The listing builds one solid part. Answer for the finished solid, in the listing's coordinates (mm). Give positions to 0.01 mm unless a question says otherwise; leave off trailing zeros. Order: outer loops, then holes, each group sorted by start corner. A loop starts at its lowest first (then second) coordinate and runs counter-clockwise, first axis right, second up.
```python
from build123d import *

# Parameters (mm, degrees)
SKETCH093_W           = 21
SKETCH093_H           = 96
EXTRUDE085_DEPTH      = 1
SKETCH140_R           = 15
EXTRUDE130_DEPTH      = 3
EXTRUDE130_DEPTH_BACK = 1
EXTRUDE074_DEPTH      = 2


with BuildPart() as cutout:
    # Sketch093 → Extrude085 (new body)
    with BuildSketch(Plane(origin=(0, 0, -25), x_dir=(1, 0, 0), z_dir=(0, 0, -1))):
        with Locations((153, -47.5)):
            Rectangle(SKETCH093_W, SKETCH093_H)
    extrude(amount=EXTRUDE085_DEPTH)


with BuildPart() as compound029:
    # Sketch140 → Extrude130 (new body, two sides)
    with BuildSketch(Plane(origin=(0, 0, -25), x_dir=(1, 0, 0), z_dir=(0, 0, -1))) as extrude130_sk:
        with Locations((25, -27)):
            Circle(SKETCH140_R)
        with Locations((103, -27)):
            Circle(SKETCH140_R)
        with Locations((64, -27)):
            Circle(SKETCH140_R)
        with Locations((103, -71)):
            Circle(SKETCH140_R)
        with Locations((25, -71)):
            Circle(SKETCH140_R)
        with Locations((64, -71)):
            Circle(SKETCH140_R)
        with Locations((188, -30)):
            Circle(SKETCH140_R)
        with Locations((231, -30)):
            Circle(SKETCH140_R)
        with Locations((188, -71)):
            Circle(SKETCH140_R)
        with Locations((231, -71)):
            Circle(SKETCH140_R)
        with Locations((284, -30)):
            Circle(SKETCH140_R)
        with Locations((329, -30)):
            Circle(SKETCH140_R)
        with Locations((284, -71)):
            Circle(SKETCH140_R)
        with Locations((329, -71)):
            Circle(SKETCH140_R)
    extrude(amount=EXTRUDE130_DEPTH)
    extrude(extrude130_sk.sketch, amount=-EXTRUDE130_DEPTH_BACK)

    # Compound029: union cutout
    add(cutout.part)


with BuildPart() as panel002:
    # Sketch082 → Extrude074 (new body)
    with BuildSketch(Plane(origin=(0, 0, -25), x_dir=(1, 0, 0), z_dir=(0, 0, -1))):
        Polygon((-2.5, 1.5), (360.5, 1.5), (360.5, -96.5), (309.5, -96.5), (309.5, -99), (257, -99), (257, -96.5), (205.5, -96.5), (205.5, -99), (153, -99), (153, -96.5), (101.5, -96.5), (101.5, -99), (49, -99), (49, -96.5), (-2.5, -96.5), align=None)
    extrude(amount=EXTRUDE074_DEPTH)

    # Cut: cut Compound029
    add(compound029.part, mode=Mode.SUBTRACT)


solid = panel002.part
```
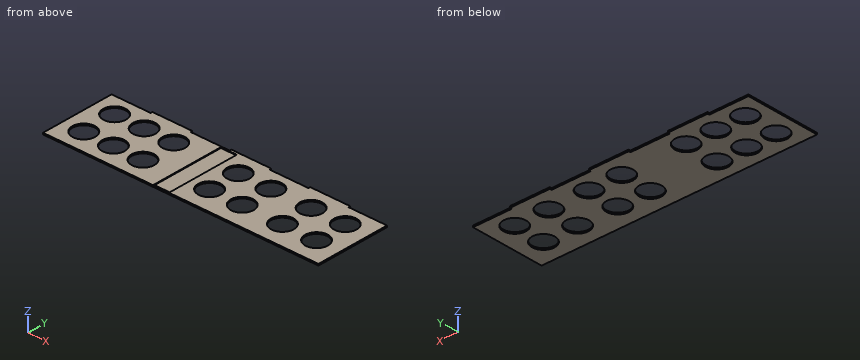
1) Find section D-D (x = 231). Write down the section's boundary in (y, z), then the cut area to 3 significant figures.
Geometry says:
outline: (-1.5, -27) - (15, -27) - (15, -25) - (-1.5, -25) - close; (45, -27) - (56, -27) - (56, -25) - (45, -25) - close; (86, -27) - (96.5, -27) - (96.5, -25) - (86, -25) - close
area: 76.0 mm2
2) Straight lines are drawn through the part: probe 1 along Y at (x, z) = (284, -26.05); probe 2 along Y at (x, z) = (231, -26.35); probe 3 along X at (y, z) = (43, -25.2). For each, find the intervals that lie inside material, in ascending order.
Geometry says:
probe 1: y = -1.5 to 15, 45 to 56, 86 to 99
probe 2: y = -1.5 to 15, 45 to 56, 86 to 96.5
probe 3: x = -2.5 to 142.5, 163.5 to 180.52, 195.48 to 223.52, 238.48 to 276.52, 291.48 to 321.52, 336.48 to 360.5
3) Find section C-C (y = 5.5). Write down the section's boundary in (x, z).
Geometry says:
outline: (-2.5, -27) - (360.5, -27) - (360.5, -25) - (163.5, -25) - (163.5, -26) - (142.5, -26) - (142.5, -25) - (-2.5, -25) - close
4) Given P1, Ø18, axis at x = 25, y = 27, coming from the -Z side, flat-ended and moving along its own axis, determine where the tip first touches the part or whether it passes through.
Geometry says:
P1: passes through
5) Find section A-A (x = 284). Write down the section's boundary in (y, z), then the cut area to 3 significant figures.
Geometry says:
outline: (-1.5, -27) - (15, -27) - (15, -25) - (-1.5, -25) - close; (45, -27) - (56, -27) - (56, -25) - (45, -25) - close; (86, -27) - (99, -27) - (99, -25) - (86, -25) - close
area: 81.0 mm2
6) Find section B-B (z = -26.5). Count the separate pieces of the cut face and the enclosed holes in it, then the cut area to 3 significant figures.
Geometry says:
separate pieces: 1
enclosed holes: 14
area: 26,100 mm2
